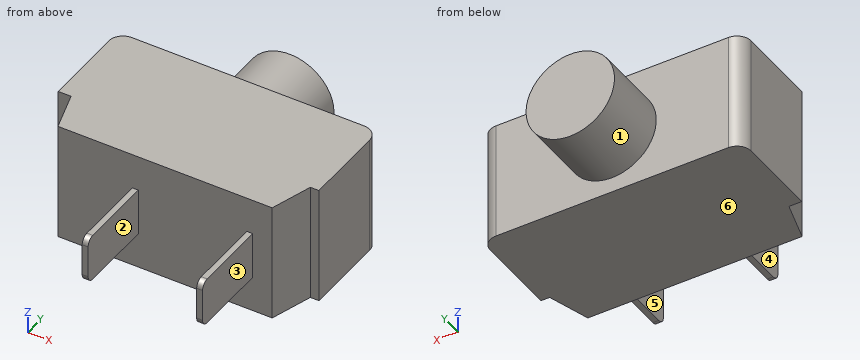
```python
from build123d import *

# Parameters (mm, degrees)
BOSS_EXTRUDE1_DEPTH = 8
FILLET1_R           = 1.905
SKETCH2_R           = 5.953125
BOSS_EXTRUDE2_DEPTH = 9.1
SKETCH1_4_W         = 0.8
SKETCH1_4_H         = 10.916687254
EXTRUDE_THIN1_DEPTH = 3.175
FILLET2_R           = 1.016


with BuildPart() as part:
    # Sketch1 → Boss-Extrude1 (new body, symmetric)
    with BuildSketch(Plane.XY):
        Polygon((-15.810469007, -12.953853844), (-17.55, -12.953853844), (-17.55, 0), (17.55, 0), (17.55, -12.953853844), (16.396875628, -12.953853844), (14.686720063, -18.5), (-14.154511139, -18.5), align=None)
    extrude(amount=BOSS_EXTRUDE1_DEPTH, both=True)

    # Fillet1
    fillet1_edges = [part.edges().sort_by_distance(p)[0] for p in [
        (-17.55, 0, 0),
        (17.55, 0, 0),
    ]]
    fillet(fillet1_edges, radius=FILLET1_R)

    # Sketch2 → Boss-Extrude2 (add)
    with BuildSketch(Plane(origin=(0, 0, 0), x_dir=(1, 0, 0), z_dir=(0, 1, 0))):
        Circle(SKETCH2_R)
    extrude(amount=BOSS_EXTRUDE2_DEPTH)

    # Sketch1_4 → Extrude-Thin1 (add, symmetric)
    with BuildSketch(Plane.XY):
        with Locations((-3.740094375, -23.958343627)):
            Rectangle(SKETCH1_4_W, SKETCH1_4_H)
        with Locations((11.66595999, -23.958343627)):
            Rectangle(SKETCH1_4_W, SKETCH1_4_H)
    extrude(amount=EXTRUDE_THIN1_DEPTH, both=True)

    # Fillet2
    fillet2_edges = [part.edges().sort_by_distance(p)[0] for p in [
        (-3.740094375, -29.416687254, 3.175),
        (-3.740094375, -29.416687254, -3.175),
        (11.66595999, -29.416687254, 3.175),
        (11.66595999, -29.416687254, -3.175),
    ]]
    fillet(fillet2_edges, radius=FILLET2_R)


solid = part.part
```
Can you work these out from the model? Positions are in its coordinate system, mm. Face numbers are marked on the shaded views. A direction names the side the tool comes from. Round coordinates to 2 decimals unless told otherwise and drop trailing zeros. Order: outer loops, then holes, each group sorted by start corner. A loop starts at its lowest first (then second) coordinate and runs counter-clockwise, first axis right, second up.
(1) If I drill on L1, parallel to X at y = -25.5, z = 0; L2, parallel to Y at x = 10, z = 0; L3, parallel to Z at x = -4, y = -21 (3 decimals), over which ranges is the centre line in solid material (lowest first)?
Results are:
L1: x = -4.14 to -3.34, 11.27 to 12.07
L2: y = -18.5 to 0
L3: z = -3.175 to 3.175
(2) We'd pull the mould along X, two halves only. Please class the marked faces 4, 5 and 6: +X half, -X half, draft (parallel to the pull), parting line (faces both ways), or undercut.
Results are:
face 4: -X half
face 5: undercut
face 6: draft
(3) If we section it at B-B (z = 0): Please give me the cut outline in (x, y) (3 decimals).
Results are:
outline: (-17.55, -12.954) - (-15.81, -12.954) - (-14.155, -18.5) - (-4.14, -18.5) - (-4.14, -29.417) - (-3.34, -29.417) - (-3.34, -18.5) - (11.266, -18.5) - (11.266, -29.417) - (12.066, -29.417) - (12.066, -18.5) - (14.687, -18.5) - (16.397, -12.954) - (17.55, -12.954) - (17.55, -1.905) arc R1.905 ccw to (15.645, 0) - (5.953, 0) - (5.953, 9.1) - (-5.953, 9.1) - (-5.953, 0) - (-15.645, 0) arc R1.905 ccw to (-17.55, -1.905) - close
(4) If we section it at C-C (x = 0): Please give me the cut outline in (y, z), plus the area to 3 significant figures.
Results are:
outline: (-18.5, -8) - (0, -8) - (0, -5.95) - (9.1, -5.95) - (9.1, 5.95) - (0, 5.95) - (0, 8) - (-18.5, 8) - close
area: 404 mm2
(5) I'm going to push flat-ended pins straight in: pin 1 (5 mm diameter, centred on y = -24.5, z = -0.5, fed in from -X); pin 2 (1 mm diameter, centred on y = 1.5, z = -1.5, fed in from +X); pin 3 (1.5 mm diameter, centred on x = -7, z = -1.5, fed in from -Y). Where does each tip first touch, or does it pass through?
Results are:
pin 1: stops at x = -4.14
pin 2: stops at x = 5.87
pin 3: stops at y = -18.5
(6) On a 3-axis mill with a long thin cutter (end or side, diameter ignored), from which of +Z, -Z, +X, -X, +Y, -Y can I reach the whole of each face in a straight line? I mean the marked faces 1, 2 and 3. Say none if no direction works.
Results are:
face 1: +Y
face 2: +Z, -Z, -Y
face 3: +Z, -Z, +X, -Y
(7) If we section it at A-A (y = -21): Please give me the cut outline in (x, z) (3 decimals), plus the area to 3 significant figures.
Results are:
outline: (-4.14, -3.175) - (-3.34, -3.175) - (-3.34, 3.175) - (-4.14, 3.175) - close; (11.266, -3.175) - (12.066, -3.175) - (12.066, 3.175) - (11.266, 3.175) - close
area: 10.2 mm2
(8) If we section it at D-D (z = -7): Please give me the cut outline in (x, y) (3 decimals), plus the area to 3 significant figures.
Results are:
outline: (-17.55, -12.954) - (-15.81, -12.954) - (-14.155, -18.5) - (14.687, -18.5) - (16.397, -12.954) - (17.55, -12.954) - (17.55, -1.905) arc R1.905 ccw to (15.645, 0) - (-15.645, 0) arc R1.905 ccw to (-17.55, -1.905) - close
area: 622 mm2
